Answer from the drawing. Dimensions are ordinates in mm from the lowest x, y and z of the part. Round coordinates to 2 decimals unless told otherwise and drop trailing zeros. Write each loop counter-clockwise with the first axis right and the second up, starting at its lowest first coordinate (ties: lowest second). Pieces come first, ordered by that corner, then holes. Notation, with made-up numbers: (-10, 18) - (37, 18) arc R22 cw to (37, 40) - close; hole circle Ø9 at (23.25, -15). An arc over 180 degrees is marked (long way). Answer in a Markdown table with one row per item.
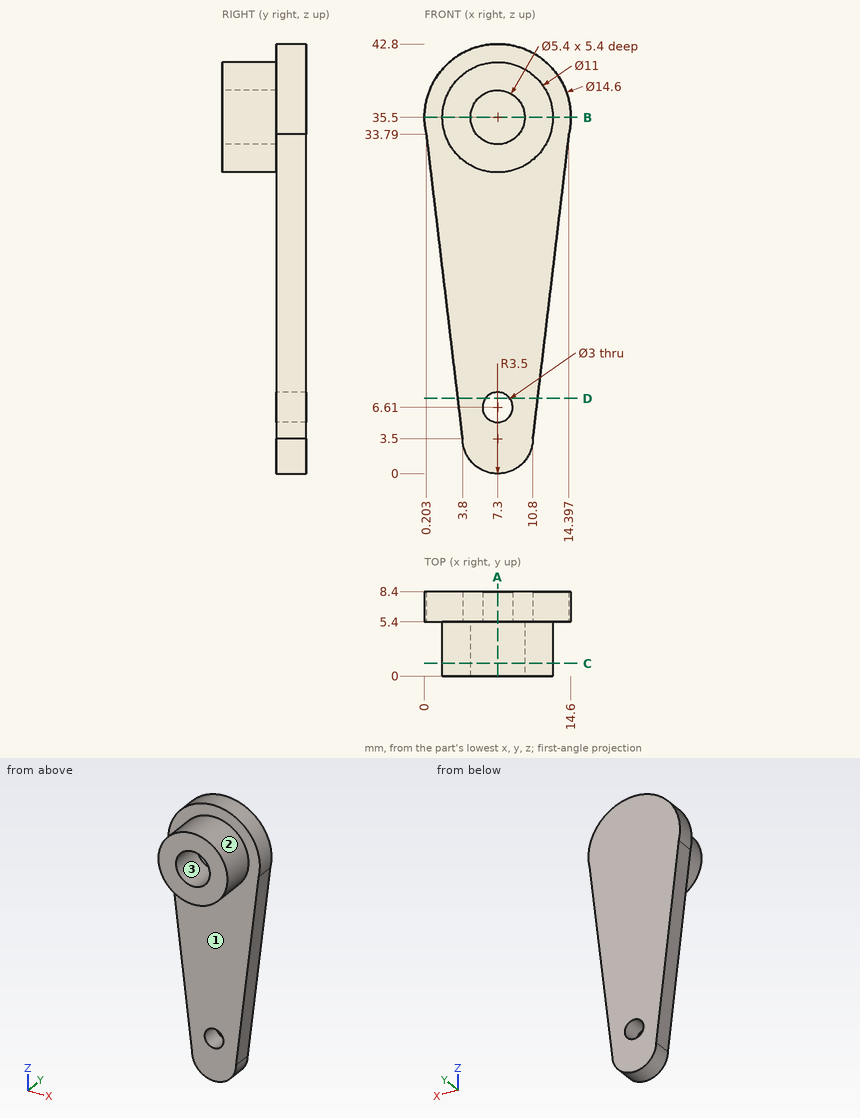
(1) Section D-D (z = 7.5) is taken. Give the vertices of the cut face in (x, y) (1 decimal), and give its area (3 significant figures).
Checked values:
| item | result |
|---|---|
| outline | (3.3, 5.4) - (6.1, 5.4) - (6.1, 8.4) - (3.3, 8.4) - close; (8.5, 5.4) - (11.3, 5.4) - (11.3, 8.4) - (8.5, 8.4) - close |
| area | 16.6 mm2 |
(2) Find the intervals of material crossed by line 1 (Z direction, x = 7.3, y = 2.75); line 2 (Y direction, x = 9.25, z = 2); line 3 (Z direction, x = 8, y = 4) (1 decimal), in increasing order.
Checked values:
| item | result |
|---|---|
| line 1 | z = 30 to 32.8, 38.2 to 41 |
| line 2 | y = 5.4 to 8.4 |
| line 3 | z = 30 to 32.9, 38.1 to 41 |
(3) Section A-A (x = 7.3) is taken. Give the vertices of the cut face in (y, z).
Checked values:
| item | result |
|---|---|
| outline | (0, 30) - (5.4, 30) - (5.4, 8.11) - (8.4, 8.11) - (8.4, 42.8) - (5.4, 42.8) - (5.4, 41) - (0, 41) - (0, 38.2) - (5.4, 38.2) - (5.4, 32.8) - (0, 32.8) - close; (5.4, 0) - (8.4, 0) - (8.4, 5.11) - (5.4, 5.11) - close |
(4) Flat-ended cylindrical pins translate along their axes: pin 1 (1.5 mm diameter, centred on x = 6, y = 3.5, fed in from +Z); pin 2 (7.5 mm diameter, centred on x = 8, z = 22.5, fed in from -Y); pin 3 (4 mm diameter, centred on x = 12, y = 2.5, fed in from -Z). Find the tip coordinate at first contact, or state that the pin passes through.
Checked values:
| item | result |
|---|---|
| pin 1 | stops at z = 40.97 |
| pin 2 | stops at y = 5.4 |
| pin 3 | stops at z = 30.71 |
(5) For a pull along X with two mould halves and no side action, classify the marked faces 1, 2 and 3 as pulls with the +X half, pulls with the -X half, needs draft (parallel to the pull), parting line crosses it, or undercut.
Checked values:
| item | result |
|---|---|
| face 1 | needs draft |
| face 2 | parting line crosses it |
| face 3 | undercut |
(6) Section C-C (y = 1.25) is taken. Give the vertices of the cut face in (x, z).
Checked values:
| item | result |
|---|---|
| outline | circle Ø11 at (7.3, 35.5); hole circle Ø5.4 at (7.3, 35.5) |
(7) Section B-B (z = 35.5) is taken. Give the vertices of the cut face in (x, y).
Checked values:
| item | result |
|---|---|
| outline | (0, 5.4) - (1.8, 5.4) - (1.8, 0) - (4.6, 0) - (4.6, 5.4) - (10, 5.4) - (10, 0) - (12.8, 0) - (12.8, 5.4) - (14.6, 5.4) - (14.6, 8.4) - (0, 8.4) - close |
